Part model, mm, in its own coordinate system. Face numbers are marked on the shaded views. Round coordinates to 2 decimals unless told otherwise and drop trailing zeros. Write each loop counter-clockwise with the first axis right and the second up, starting at its lowest first coordinate (ties: lowest second). Pieces come first, ordered by that corner, then holes.
Autodesk Inventor part; units mm, degrees
ref_plane "YZ Plane" through (0, 0, 0) normal (1, 0, 0) x (0, 1, 0)
ref_plane "XZ Plane" through (0, 0, 0) normal (0, 1, 0) x (-1, 0, 0)
ref_plane "XY Plane" through (0, 0, 0) normal (0, 0, 1) x (1, 0, 0)
sketch "Sketch1" plane through (0, 0, 0) normal (0, 1, 0) x (-1, 0, 0)
  line L0 (-85.5, -44.5) -> (85.5, -44.5)
  line L1 (85.5, -44.5) -> (85.5, 44.5)
  line L2 (85.5, 44.5) -> (-85.5, 44.5)
  line L3 (-85.5, 44.5) -> (-85.5, -44.5)
  line L4 (-85.5, -44.5) -> (85.5, 44.5) construction
  line L5 (85.5, -44.5) -> (-85.5, 44.5) construction
  line L6 (-81, -38.5) -> (81, -38.5)
  line L7 (81, -38.5) -> (81, 38.5)
  line L8 (81, 38.5) -> (-81, 38.5)
  line L9 (-81, 38.5) -> (-81, -38.5)
  line L10 (-81, -38.5) -> (81, 38.5) construction
  line L11 (81, -38.5) -> (-81, 38.5) construction
  line L12 (81, 38.5) -> (79.55, 38.5)
  line L13 (81, 37.05) -> (81, 38.5)
  circle A0 centre (79.55, 37.05) radius 1.45
  circle A1 centre (79.55, -37.05) radius 1.45
  circle A2 centre (-79.55, -37.05) radius 1.45
  circle A3 centre (-79.55, 37.05) radius 1.45
  line L14 (81, 38.5) -> (78.1, 38.5)
  line L15 (78.1, 38.5) -> (78.1, 35.6)
  line L16 (78.1, 35.6) -> (81, 35.6)
  line L17 (81, 35.6) -> (81, 38.5)
  line L18 (81, 38.5) -> (78.1, 35.6) construction
  line L19 (78.1, 38.5) -> (81, 35.6) construction
  line L20 (81, -35.6) -> (78.1, -35.6)
  line L21 (78.1, -35.6) -> (78.1, -38.5)
  line L22 (78.1, -38.5) -> (81, -38.5)
  line L23 (81, -38.5) -> (81, -35.6)
  line L24 (81, -35.6) -> (78.1, -38.5) construction
  line L25 (78.1, -35.6) -> (81, -38.5) construction
  line L26 (-81, -38.5) -> (-78.1, -38.5)
  line L27 (-78.1, -35.6) -> (-81, -38.5) construction
  line L28 (-81, -35.6) -> (-78.1, -38.5) construction
  line L29 (-78.1, 38.5) -> (-81, 38.5)
  line L30 (-81, 38.5) -> (-81, 35.6)
  line L31 (-78.1, 38.5) -> (-81, 35.6) construction
  line L32 (-81, 38.5) -> (-78.1, 35.6) construction
  circle A4 centre (-79.55, 37.05) radius 2.5
  line L33 (-95.5566, 0) -> (75.4434, 0)
  line L34 (0, 31.9167) -> (0, -57.0833)
  circle A5 centre (-79.55, -37.05) radius 2.5
  circle A6 centre (79.55, 37.05) radius 2.5
  circle A7 centre (79.55, -37.05) radius 2.5
  line L35 (140, 0) -> (-140, 0)
  line L36 (0, -112) -> (0, 112)
  line L37 (-100, 59.2475) -> (100, 59.2475)
  line L38 (100, 59.2475) -> (100, -59.2475)
  line L39 (100, -59.2475) -> (-100, -59.2475)
  line L40 (-100, -59.2475) -> (-100, 59.2475)
  line L41 (-100, 59.2475) -> (100, -59.2475) construction
  line L42 (100, 59.2475) -> (-100, -59.2475) construction
  line L43 (-100, 80) -> (-20, 80)
  line L44 (-20, 80) -> (-20, -80)
  line L45 (-20, -80) -> (-100, -80)
  line L46 (-100, -80) -> (-100, 80)
  line L47 (-100, 80) -> (-20, -80) construction
  line L48 (-20, 80) -> (-100, -80) construction
  point P0 (0, 0)
  point P1 (-79.55, 38.5)
  point P2 (-81, 37.05)
  point P3 (-81, -37.05)
  point P4 (-79.55, -38.5)
  point P5 (79.55, -38.5)
  point P6 (81, -37.05)
  point P7 (-60, 0)
  point P8 (-20, 59.2475)
  point P9 (-20, -59.2475)
  dimension "d0" = 171
  dimension "d1" = 89
  dimension "d2" = 162
  dimension "d3" = 77
  dimension "d7" = 2.9
  dimension "d8" = 2.9
  dimension "d9" = 2.9
  dimension "d10" = 2.9
  dimension "d53" = 5
  dimension "d56" = 200
  dimension "d57" = 80
  dimension "d58" = 160
extrude "Extrusion1" add sketch "Sketch1" along normal blind 55 contours A2 | A3 | A1 | A0
extrude "Extrusion2" add sketch "Sketch1" along normal blind 4 contours L44 L33 L34 L6 | L6 A5 L9 L33 L44 | L9 A4 L8 L44 L33 | L34 L33 L35 L7 A7 L6 | L6 A2 L9 A5 | L44 L8 L36 L34 L33 | L9 A3 L8 A4 | A7 L7 L20 L21 L6 | L34 L36 L8 A6 L7 L35 L33 | L21 A1 L6 | A6 L8 L15 L16 L7 | L21 L20 A1 | L7 A1 L20 | L16 A0 L7 | L8 A0 L15 | L16 L15 A0
extrude "Extrusion3" add sketch "Sketch1" along normal blind 25 contours L3 L33 L9 A5 L6 L44 L0 | L44 L6 L34 L0 | L3 L2 L44 L8 A4 L9 L33 | L34 L6 A7 L7 L35 L1 L0 | A5 L9 L6 | L2 L36 L8 L44 | A4 L8 L9 | L35 L7 A6 L8 L36 L2 L1 | L6 L7 A7 | L7 L8 A6
chamfer "Chamfer1" distance 2 angle 45 4 edges at (0, 25, 44.5) (85.5, 25, 0) (0, 25, -44.5) (-85.5, 25, 0)
fillet "Fillet6" radius 2 1 edges at (85.5, 11.5, 44.5)
fillet "Fillet7" radius 2 1 edges at (85.5, 11.5, -44.5)
fillet "Fillet8" radius 2 1 edges at (-85.5, 11.5, 44.5)
fillet "Fillet9" radius 2 1 edges at (-85.5, 11.5, -44.5)
extrude "Extrusion11" add sketch "Sketch1" along normal blind 45 contours A5 L9 L6 | L6 A2 L9 A5 | A4 L8 L9 | L9 A3 L8 A4 | A7 L7 L20 L21 L6 | L6 L7 A7 | A2 L6 L9 | A2 | L21 A1 L6 | L9 L8 A3 | A3 | A6 L8 L15 L16 L7 | L7 L8 A6 | A1 L7 L6 | A1 | L21 L20 A1 | L7 A1 L20 | L16 A0 L7 | L8 A0 L15 | A0 L8 L7 | A0 | L16 L15 A0
extrude "Extrusion12" add sketch "Sketch1" along normal blind 10 contours L0 L44 L39 L40 L35 L33 L3 | L0 L34 L36 L39 L44 | L33 L35 L40 L37 L44 L2 L3 | L0 L1 L35 L38 L39 L36 L34 | L44 L45 L46 L39 | L44 L37 L36 L2 | L1 L2 L36 L37 L38 L35 | L37 L46 L43 L44
chamfer "Chamfer2" distance 2 angle 45 8 edges at (100, 10, 0) (60, 10, 80) (20, 10, 69.6238) (60, 10, -80) (20, 10, -69.6238) (-40, 10, -59.2475) (-40, 10, 59.2475) (-100, 10, 0)
sketch "Sketch4" plane through (0, 0, 0) normal (0, -1, 0) x (1, 0, 0)
  circle A0 centre (-11.2675, 0) radius 2
  circle A1 centre (-71.2675, 0) radius 2
  circle A2 centre (-41.2675, 30) radius 2
  circle A3 centre (-11.2675, 0) radius 1.9
  circle A4 centre (-71.2675, 0) radius 1.9
  circle A5 centre (-41.2675, 30) radius 1.9
  point P0 (0, 0)
  dimension "d64" = 3.8
extrude "Extrusion13" add sketch "Sketch4" along normal blind 10 contours A3 | A4 | A5
properties part number "Buggy_Body_Wheel_Wells"
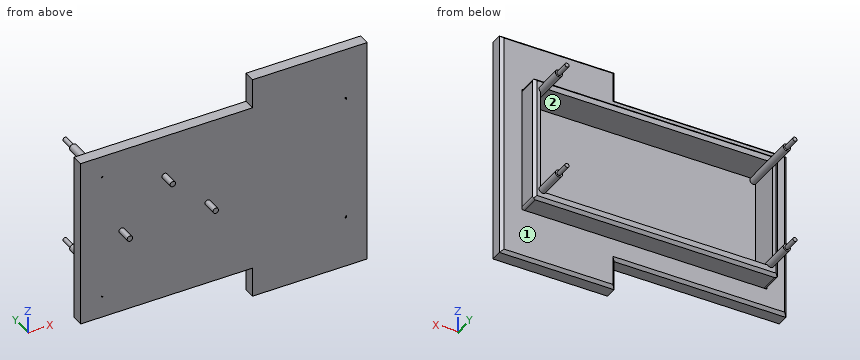
Q1. Cut at C-C on x = 3. Write the cut outline in (y, z), plus the area to 3 significant figures.
Values follow:
outline: (0, -59.25) - (8, -59.25) - (10, -57.25) - (10, -44.5) - (23, -44.5) - (25, -42.5) - (25, -38.5) - (4, -38.5) - (4, 38.5) - (25, 38.5) - (25, 42.5) - (23, 44.5) - (10, 44.5) - (10, 57.25) - (8, 59.25) - (0, 59.25) - close
area: 895 mm2
Q2. Mould opens along X. For the marked faces 1 and 2 say: +X half, -X half, draft (parallel to the pull), parting line (faces both ways), or undercut.
Values follow:
face 1: draft
face 2: undercut
Q3. Wall check: L1, parallel to Z at x = -34, y = 5; L2, parallel to X at y = 7.5, z = -21.5; L3, parallel to Y at x = 60, z = -9. Give the ranges that are in metal, low to high.
Values follow:
L1: z = -59.25 to -38.5, 38.5 to 59.25
L2: x = -100 to -81, 81 to 100
L3: y = 0 to 4
Q4. Cut at A-A on x = 32. Write the cut outline in (y, z).
Values follow:
outline: (0, -80) - (8, -80) - (10, -78) - (10, -44.5) - (23, -44.5) - (25, -42.5) - (25, -38.5) - (4, -38.5) - (4, 38.5) - (25, 38.5) - (25, 42.5) - (23, 44.5) - (10, 44.5) - (10, 78) - (8, 80) - (0, 80) - close
Q5. Cut at B-B on z = -64. Write the cut outline in (x, y).
Values follow:
outline: (20, 0) - (100, 0) - (100, 8) - (98, 10) - (22, 10) - (20, 8) - close
Q6. Drop flat-ended pins along their axis: pin 1 (1 mm diameter, centred on x = 43.5, y = 24.5, fed in from -Z); pin 2 (3 mm diameter, centred on x = -67, z = -9, fed in from -Y); pin 3 (8 mm diameter, centred on x = -12.5, z = 33, fed in from +Y); pin 4 (10 mm diameter, centred on y = 37, z = 49, fed in from +X). Give the stop position or say it passes through.
Values follow:
pin 1: stops at z = -43.5
pin 2: stops at y = 0
pin 3: stops at y = 4
pin 4: passes through
Q7. Cut at D-D on z = 48. Write the cut outline in (x, y).
Values follow:
outline: (-100, 0) - (100, 0) - (100, 8) - (98, 10) - (-98, 10) - (-100, 8) - close
